The listing builds one solid part. Answer for the finished solid, in the listing's coordinates (mm). Face numbers are marked on the shaded views. A direction names the side the tool comes from. Round coordinates to 2 decimals unless told otherwise and drop trailing zeros. Write each loop counter-clockwise with the first axis right and the second up, starting at its lowest first coordinate (ties: lowest second). Pieces come first, ordered by that corner, then holes.
(1) A cutting plane is placed at A-A, the plane x = 50. Give the vertices of the cut face in (y, z), and give its area (3 significant figures).
(2) A cutting plane is placed at C-C, the plane y = 42. Give the vertices of the cut face in (x, z).
(3) For the marked faces 1 and 2, determine the directions among +Z, -Z, +X, -X, +Y, -Y from which every point of the face is accessible in a straight line to the end or side of a thin tool.
(4) A cutting plane is placed at B-B, the plane z = -50. Give the vertices of the cut face in (x, y), and give its area (3 significant figures).
(5) A cutting plane is placed at D-D, the plane x = 86. Give the vertices of the cut face in (y, z), and give its area (3 significant figures).
(6) Each of these flat-tipped pins is pushed along its axis until it touches: pin 1 Ø3 at (x, y) = (26, 64.5) entering from -Z; pin 2 Ø5.5 at (x, y) = (84.91, 37) entering from -Z; pin 3 Ø12 at (x, z) = (40.5, -37.5) entering from +Y. Where does it stop, or does it pass through?
(7) Find the intervals of material crossed by probe 1 along Z at (x, y) = (50, 7); probe 2 along Y at (x, z) = (73, -66); probe 3 along Z at (x, y) = (74, 37), in increasing order.
from build123d import *

# Parameters (mm, degrees)
F1_DEPTH = 100
F2_R     = 3.332982
F3_DEPTH = 25
F4_R     = 3.762858
F5_DEPTH = 25


with BuildPart() as f1:
    # F0 (on Right) → F1 (new body)
    with BuildSketch(Plane.YZ):
        with BuildLine():
            Line((80, 0), (0, 0))
            Line((0, 0), (0, -100))
            Line((0, -100), (9.5, -100))
            Line((9.5, -100), (9.5, -15.5))
            ThreePointArc((9.5, -15.5), (11.257359, -11.257359), (15.5, -9.5))
            Line((15.5, -9.5), (80, -9.5))
            Line((80, -9.5), (80, 0))
        make_face()
    extrude(amount=F1_DEPTH)

    # F2 (on face) → F3 (cut)
    with BuildSketch(Plane.XY):
        with Locations((84.909265, 36.999489)):
            Circle(F2_R)
        with BuildLine():
            ThreePointArc((5.484932, 33.531748), (10.176936, 29.232318), (14.476366, 33.924322))
            ThreePointArc((14.476366, 33.924322), (14.426042, 35.46154), (14.409265, 36.999489))
            ThreePointArc((14.409265, 36.999489), (14.426042, 38.537438), (14.476366, 40.074656))
            ThreePointArc((14.476366, 40.074656), (10.176936, 44.76666), (5.484932, 40.46723))
            ThreePointArc((5.484932, 40.46723), (5.428184, 38.733772), (5.409265, 36.999489))
            ThreePointArc((5.409265, 36.999489), (5.428184, 35.265206), (5.484932, 33.531748))
        make_face()
    extrude(amount=-F3_DEPTH, mode=Mode.SUBTRACT)

    # F4 (on face) → F5 (cut)
    with BuildSketch(Plane.XZ):
        with Locations((50, -50)):
            Circle(F4_R)
    extrude(amount=-F5_DEPTH, mode=Mode.SUBTRACT)


solid = f1.part
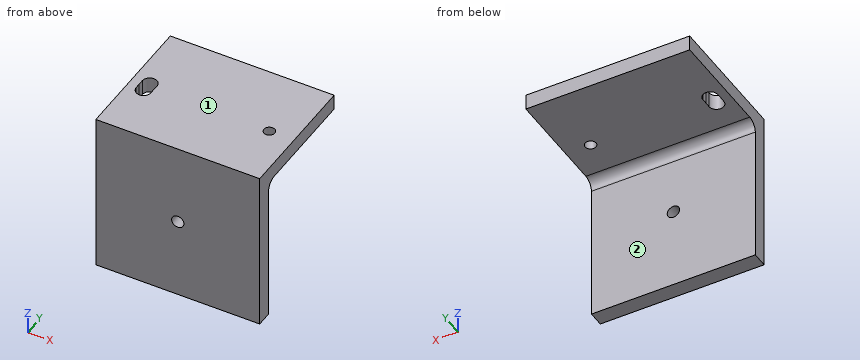
Solutions:
1. outline: (0, -100) - (9.5, -100) - (9.5, -53.76) - (0, -53.76) - close; (0, -46.24) - (9.5, -46.24) - (9.5, -15.5) arc R6 cw to (15.5, -9.5) - (80, -9.5) - (80, 0) - (0, 0) - close
1. area: 1,560 mm2
2. outline: (0, -9.5) - (5.83, -9.5) - (5.83, 0) - (0, 0) - close; (14.14, -9.5) - (100, -9.5) - (100, 0) - (14.14, 0) - close
3. face 1: +Z, +X, -X, +Y, -Y
3. face 2: -Z, +X, -X, +Y
4. outline: (0, 0) - (46.24, 0) - (46.24, 9.5) - (0, 9.5) - close; (53.76, 0) - (100, 0) - (100, 9.5) - (53.76, 9.5) - close
4. area: 879 mm2
5. outline: (0, -100) - (9.5, -100) - (9.5, -15.5) arc R6 cw to (15.5, -9.5) - (33.85, -9.5) - (33.85, 0) - (0, 0) - close; (40.15, -9.5) - (80, -9.5) - (80, 0) - (40.15, 0) - close
5. area: 1,570 mm2
6. pin 1: stops at z = -9.5
6. pin 2: passes through
6. pin 3: stops at y = 9.5
7. probe 1: z = -100 to -53.76, -46.24 to 0
7. probe 2: y = 0 to 9.5
7. probe 3: z = -9.5 to 0
